Source: CAD feature listing. Evaluate the final solid. Frame: model axes, mm. Give positions to 0.01 mm unless a question says otherwise; leave off trailing zeros. Loops run counter-clockwise (first coordinate to the right, second up) from the corner with the lowest first, then second, coordinate; pieces in that order, holes last. Notation, with made-up numbers: M 85,64.5 L 94,64.5 A9 ccw 94,76.5 Z; hole C -2.5,86 d3. An arc over 180 degrees is marked long. Answer in a Markdown table with one row per item.
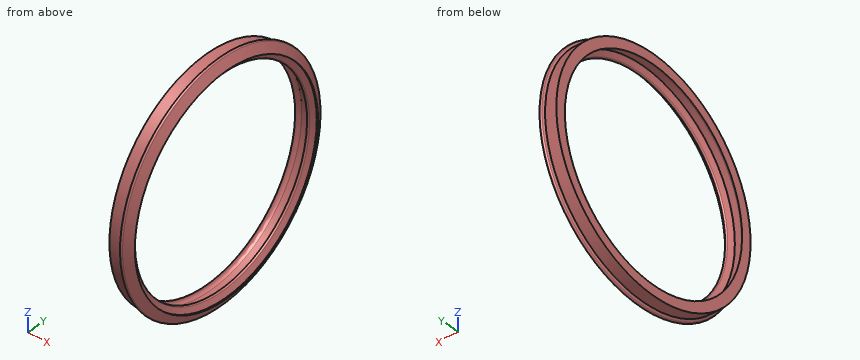
```python
from build123d import *


with BuildPart() as part:
    # Эскиз1 → Повернуть1 (revolve)
    with BuildSketch(Plane.XY, mode=Mode.PRIVATE) as revolve_1_sk:
        with BuildLine():
            Line((0, 15.9), (1.553589838, 15.9))
            Line((1.553589838, 15.9), (1.726794919, 16.2))
            ThreePointArc((1.726794919, 16.2), (1.9, 16.3), (2.073205081, 16.2))
            Line((2.073205081, 16.2), (2.766025404, 15))
            Line((2.766025404, 15), (2.577350269, 15))
            Line((2.577350269, 15), (2.173205081, 14.3))
            ThreePointArc((2.173205081, 14.3), (2, 14.2), (1.826794919, 14.3))
            Line((1.826794919, 14.3), (1.422649731, 15))
            Line((1.422649731, 15), (0, 15))
            Line((0, 15), (0, 15.9))
        make_face()
    revolve(revolve_1_sk.sketch.rotate(Axis((0, 0, 0), (1, 0, 0)), 90), axis=Axis((0, 0, 0), (1, 0, 0)))

    # Эскиз2 → Повернуть2 (revolve)
    with BuildSketch(Plane.XY, mode=Mode.PRIVATE) as revolve_2_sk:
        with BuildLine():
            Line((0, 14.5), (0, 15))
            Line((0, 15), (0.5, 15))
            ThreePointArc((0.5, 15), (0.146446609, 14.853553391), (0, 14.5))
        make_face()
    revolve(revolve_2_sk.sketch.rotate(Axis((0, 0, 0), (1, 0, 0)), 90), axis=Axis((0, 0, 0), (1, 0, 0)))


solid = part.part
```
1) Material intervals for L1, parallel to Y at x = 1.15, z = 0; L2, parallel to Y at x = 2.65, z = 0; L3, parallel to Z at x = 0.2, y = 12, sorted ascending.
Reply:
| item | result |
|---|---|
| L1 | y = -15.9 to -15, 15 to 15.9 |
| L2 | y = -15.2 to -15, 15 to 15.2 |
| L3 | z = -10.43 to -8.83, 8.83 to 10.43 |
2) Section A-A, the plane y = 0. Return loops of the section in (x, z).
Reply:
| item | result |
|---|---|
| outline | M 0,-15.9 L 1.55,-15.9 L 1.73,-16.2 A0.2 ccw 2.07,-16.2 L 2.77,-15 L 2.58,-15 L 2.17,-14.3 A0.2 ccw 1.83,-14.3 L 1.42,-15 L 0.5,-15 A0.5 cw 0,-14.5 Z; M 0,14.5 A0.5 cw 0.5,15 L 1.42,15 L 1.83,14.3 A0.2 ccw 2.17,14.3 L 2.58,15 L 2.77,15 L 2.07,16.2 A0.2 ccw 1.73,16.2 L 1.55,15.9 L 0,15.9 Z |
3) Pin query (flat end, axial travel): pin 1 Ø1 at (x, y) = (2, 1) entering from +Z; pin 2 Ø1.5 at (x, y) = (2.5, -6.5) entering from -Z. Return the tip coordinate at first contact, or that it passes through.
Reply:
| item | result |
|---|---|
| pin 1 | stops at z = 16.29 |
| pin 2 | stops at z = -15.15 |
